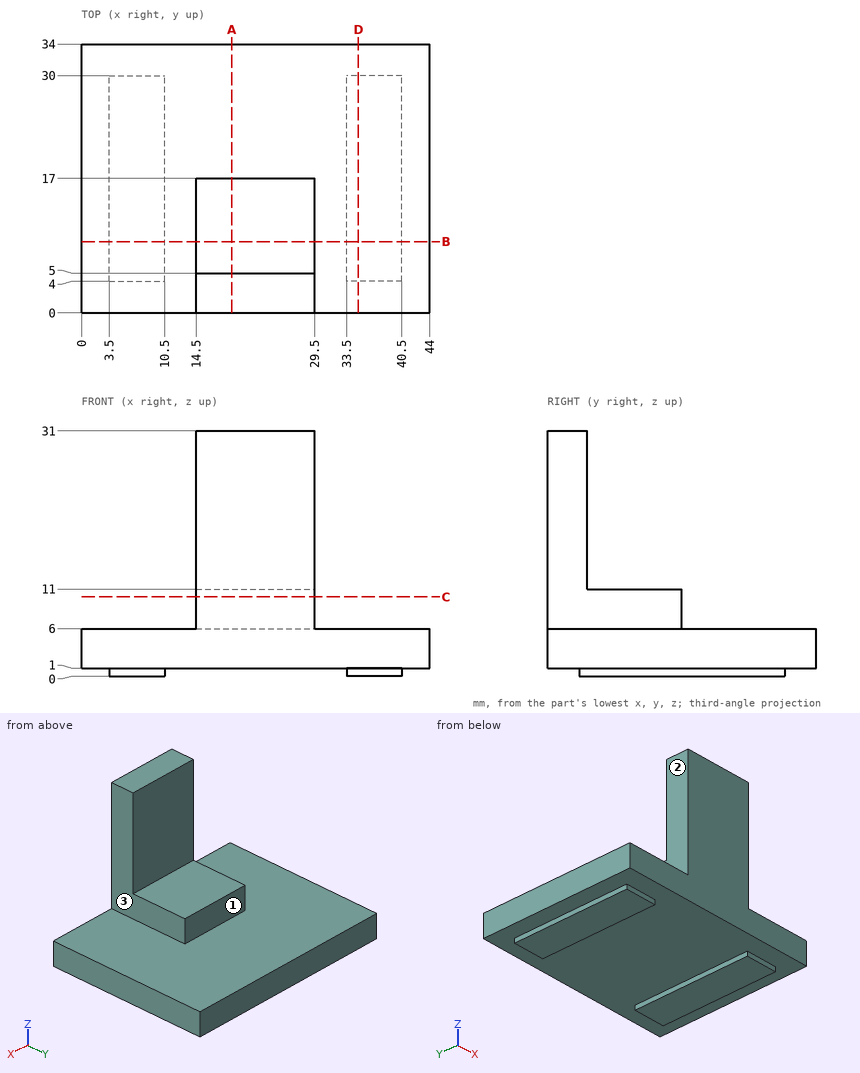
Geometry check sheet. Reference: drawing and pictorial views, mm from the part's lowest x, y, z. A direction names the side the tool comes from. Round coordinates to 2 decimals unless told otherwise and drop trailing zeros. Write each loop counter-clockwise with the first axis right and the second up, starting at its lowest first coordinate (ties: lowest second). Pieces come first, ordered by that corner, then holes.
Item 1: Material ranges on line 1 along X through (y, z) = (4, 28.5); line 2 along Z through (x, y) = (37, 17); line 3 along Z through (x, y) = (17.5, 5.5), recorded low to high.
Determined:
line 1: x = 14.5 to 29.5
line 2: z = 0 to 6
line 3: z = 1 to 11
Item 2: Section check C-C (z = 10). Record the boundary of the cut face in (x, y).
Determined:
outline: (14.5, 0) - (29.5, 0) - (29.5, 17) - (14.5, 17) - close
Item 3: Go/stop test with flat-tipped pins: pin 1 Ø0.8 at (y, z) = (17.5, 0.5) entering from -X; pin 2 Ø0.8 at (y, z) = (12.5, 0.5) entering from +X; pin 3 Ø1 at (y, z) = (13.5, 8.5) entering from +X; pin 4 Ø1.5 at (x, z) = (31, 26) entering from -Y. Record where each tip stops, or that it passes through.
Determined:
pin 1: stops at x = 3.5
pin 2: stops at x = 40.5
pin 3: stops at x = 29.5
pin 4: passes through
Item 4: Section check D-D (x = 35). Record the boundary of the cut face in (y, z), plus the area to 3 significant figures.
Determined:
outline: (0, 1) - (4, 1) - (4, 0) - (30, 0) - (30, 1) - (34, 1) - (34, 6) - (0, 6) - close
area: 196 mm2
Item 5: Section check B-B (y = 9). Record the boundary of the cut face in (x, z).
Determined:
outline: (0, 1) - (3.5, 1) - (3.5, 0) - (10.5, 0) - (10.5, 1) - (33.5, 1) - (33.5, 0) - (40.5, 0) - (40.5, 1) - (44, 1) - (44, 6) - (29.5, 6) - (29.5, 11) - (14.5, 11) - (14.5, 6) - (0, 6) - close
Item 6: Access from +Z, -Z, +X, -X, +Y, -Y to the whole of each face (thin tool, end or side, straight path). Record for the marked faces 1, 2 and 3.
Determined:
face 1: +Z, +X, -X, +Y
face 2: +Z, -X, +Y, -Y
face 3: +Z, +X, +Y, -Y
Item 7: Section check A-A (x = 19). Record the boundary of the cut face in (y, z), plus the area to 3 significant figures.
Determined:
outline: (0, 1) - (34, 1) - (34, 6) - (17, 6) - (17, 11) - (5, 11) - (5, 31) - (0, 31) - close
area: 355 mm2
